from build123d import *

# Parameters (mm, degrees)
F1_DEPTH  = 17.78
F2_W      = 7.62
F2_H      = 17.78
F3_DEPTH  = 16.51
F4_SIZE   = 6.35
F5_R      = 2.65
F6_DEPTH  = 25.4
F7_R      = 5.08
F12_DEPTH = 17.78
F13_R     = 8.3185
F14_DEPTH = 17.781


# Not quite as in the source:
# - two fillets or chamfers of one size are made in one step
# - a feature names something its author has since deleted; it is built from what else it names


with BuildPart() as f1:
    # F0 (on Top) → F1 (new body)
    with BuildSketch(Plane.XY):
        Polygon((0, 12.7), (0, -12.7), (17.78, -12.7), (17.78, 5.08), (10.16, 12.7), align=None)
    extrude(amount=F1_DEPTH)

    # F2 (on face) → F3 (join)
    with BuildSketch(Plane.YZ.offset(17.78)):
        with Locations((1.27, 8.89)):
            Rectangle(F2_W, F2_H)
    extrude(amount=F3_DEPTH)

    # F4
    f4_edges = [f1.edges().sort_by_distance(p)[0] for p in [
        (34.29, 1.27, 17.78),
    ]]
    chamfer(f4_edges, length=F4_SIZE)

    # F5 (on face) → F6 (cut)
    with BuildSketch(Plane.XZ.offset(2.54)):
        with Locations((27.305, 6.35)):
            Circle(F5_R)
    extrude(amount=-F6_DEPTH, mode=Mode.SUBTRACT)

    # F7
    f7_edges = [f1.edges().sort_by_distance(p)[0] for p in [
        (27.94, 1.27, 17.78),
        (34.29, 1.27, 11.43),
        (17.78, -12.7, 8.89),
        (17.78, 5.08, 8.89),
        (10.16, 12.7, 8.89),
        (34.29, 1.27, 0),
    ]]
    fillet(f7_edges, radius=F7_R)

    # F11 (on face) → F12 (join, through all)
    with BuildSketch(Plane.XY.offset(17.78)):
        with BuildLine():
            Line((0, -12.7), (0, 12.7))
            ThreePointArc((0, 12.7), (-12.7, 0), (0, -12.7))
        make_face()
    extrude(amount=-F12_DEPTH)

    # F13 (on face) → F14 (cut, through all)
    with BuildSketch(Plane.XY.offset(17.78)):
        Circle(F13_R)
    extrude(amount=-F14_DEPTH, mode=Mode.SUBTRACT)


solid = f1.part
Geometry check sheet. Reference: the model listing, model coordinates, mm. A direction names the side the tool comes from. Give positions to 0.01 mm unless a question says otherwise; leave off trailing zeros. Write each loop counter-clockwise with the first axis right and the second up, starting at its lowest first coordinate (ties: lowest second). Pieces come first, ordered by that corner, then holes.
1) Cross-section at A-A (y = 0). Count the separate pieces of the cut face and the enclosed holes in it, plus the area to 3 significant figures.
Values follow:
separate pieces: 2
enclosed holes: 1
area: 491 mm2
2) Cross-section at D-D (y = -3.25). Record the boundary of the cut face in (x, z), plus the area to 3 significant figures.
Values follow:
outline: (-12.28, 0) - (-7.66, 0) - (-7.66, 17.78) - (-12.28, 17.78) - close; (7.66, 0) - (17.78, 0) - (17.78, 17.78) - (7.66, 17.78) - close
area: 262 mm2
3) Release check for a two-part mould opening along X. For faces 1 (the face through (-12.697, 0.279, 9.014)), 2 (the face through (-1.08, 8.25, 9.01)), 3 (the face through (17.966, 5.456, 9.014)) record: released by +X, released by -X, zero draft, split by the parting line, or undercut.
Values follow:
face 1: released by -X
face 2: undercut
face 3: released by +X
4) Cross-section at B-B (z = 6.35). Record the boundary of the cut face in (x, y) (1 decimal).
Values follow:
outline: (0, -12.7) - (12.7, -12.7) arc R5.1 ccw to (17.8, -7.6) - (17.8, -2.5) - (24.7, -2.5) - (24.7, 5.1) - (19.9, 5.1) arc R5.1 cw to (16.3, 6.6) - (11.6, 11.2) arc R5.1 ccw to (8.1, 12.7) - (0, 12.7) arc R12.7 ccw to start; (30, -2.5) - (34.3, -2.5) - (34.3, 5.1) - (30, 5.1) - close; hole circle Ø16.6 at (0, 0)
5) Go/stop test with flat-tipped pins: pin 1 Ø1.5 at (x, y) = (27.5, -3) entering from -Z; pin 2 Ø2 at (y, z) = (2.5, 6) entering from -X; pin 3 Ø10 at (y, z) = (7, 8) entering from -X; pin 4 Ø8.5 at (x, z) = (27.305, 6.35) entering from +Y. Record where each tip stops, or that it passes through.
Values follow:
pin 1: stops at z = 0
pin 2: stops at x = -12.61
pin 3: stops at x = -12.54
pin 4: stops at y = 5.08
6) Set-up check for faces 4 (the face through (27.754, 1.323, 17.404)), 5 (the face through (26, -2.54, 9)), 6 (the face through (25, 5.08, 9)): record each of +Z, -Z, +X, -X, +Y, -Y from which the full face is reachable in a straight line by a thin tool's end or side.
Values follow:
face 4: +Z, +X, +Y, -Y
face 5: +Z, -Z, +X, -Y
face 6: +Z, -Z, +X, +Y
7) Thickness scan on line 1 (Y direction, x = 0, z = 13.75); line 2 (X direction, y = 3, z = 15.5); line 3 (X direction, y = 1.25, z = 4.75). Record the ranges inside material, lowest first.
Values follow:
line 1: y = -12.7 to -8.32, 8.32 to 12.7
line 2: x = -12.34 to -7.76, 7.76 to 30.22
line 3: x = -12.64 to -8.22, 8.22 to 25.19, 29.42 to 34.28
8) Cross-section at C-C (x = 6). Record the boundary of the cut face in (y, z).
Values follow:
outline: (-12.7, 0) - (-5.76, 0) - (-5.76, 17.78) - (-12.7, 17.78) - close; (5.76, 0) - (12.7, 0) - (12.7, 17.78) - (5.76, 17.78) - close
